Model file for the job. Use its own axes, mm. Coordinates: 2 decimals unless noted, no trailing zeros. Write each loop counter-clockwise with the first axis right and the second up, starting at its lowest first coordinate (ties: lowest second). Pieces come first, ordered by that corner, then holes. Notation, with made-up numbers: M 45,80 L 73,80 A23 ccw 73,91 Z; hole C 48.5,-38.5 d5. An arc over 180 degrees is marked long. Put each result on its own line as item: value. Start each with the question number.
Q1. Cut at A-A (y = 15). Write the cut outline in (x, z), then the cut area to 3 significant figures.
Q2. Cut at C-C (x = -7.75). Write the cut outline in (y, z), then the cut area to 3 significant figures.
Q3. Drill centre lines: line 1 along Z through (x, y) = (0.75, 28); line 2 along Z through (x, y) = (-5, 13.5); line 3 along X through (y, z) = (8.5, 35). Where is each one in solid material? Low to high.
Q4. Pull direction X, two halves, no side cores. Call faces 1 (the cylindrical face through (2.4, 15.2, 38.2)), 2 (the flat face through (0, 0, -1)), 3 (the flat face through (15, 15, 1)): pulls with the +X half, pulls with the -X half, needs draft (parallel to the pull), parting line crosses it, or undercut.
Q5. Cut at D-D (x = 2.5). Write the cut outline in (y, z), then the cut area to 3 significant figures.
Q6. Cut at B-B (z = -20). Write the cut outline in (x, y).
```python
from build123d import *

# Parameters (mm, degrees)
SKETCH1_W           = 30
SKETCH1_H           = 90
BOSS_EXTRUDE1_DEPTH = 30
SKETCH2_R           = 4
CUT_EXTRUDE1_DEPTH  = 62.846584384
SKETCH3_R           = 4
CUT_EXTRUDE2_DEPTH  = 57.124860802


with BuildPart() as part:
    # Sketch1 → Boss-Extrude1 (new body)
    with BuildSketch(Plane(origin=(0, 0, 0), x_dir=(1, 0, 0), z_dir=(0, 1, 0))):
        Rectangle(SKETCH1_W, SKETCH1_H)
    extrude(amount=BOSS_EXTRUDE1_DEPTH)

    # Sketch2 → Cut-Extrude1 (cut, through all)
    with BuildSketch(Plane.ZY.offset(15)):
        with Locations((-20, 15)):
            Circle(SKETCH2_R)
        with Locations((20, 15)):
            Circle(SKETCH2_R)
    extrude(amount=-CUT_EXTRUDE1_DEPTH, mode=Mode.SUBTRACT)

    # Sketch3 → Cut-Extrude2 (cut, through all)
    with BuildSketch(Plane(origin=(0, 30, 0), x_dir=(1, 0, 0), z_dir=(0, 1, 0))):
        with Locations(Location((0, 35, 0), (0, 0, 270))):
            Circle(SKETCH3_R)
        with Locations(Location((0, -35, 0), (0, 0, 90))):
            Circle(SKETCH3_R)
    extrude(amount=-CUT_EXTRUDE2_DEPTH, mode=Mode.SUBTRACT)


solid = part.part
```
Computed values:
1. outline: M -15,-45 L 15,-45 L 15,-24 L -15,-24 Z; M -15,-16 L 15,-16 L 15,16 L -15,16 Z; M -15,24 L 15,24 L 15,45 L -15,45 Z; hole C 0,-35 d8; hole C 0,35 d8
1. area: 2,120 mm2
2. outline: M 0,-45 L 30,-45 L 30,45 L 0,45 Z; hole C 15,-20 d8; hole C 15,20 d8
2. area: 2,600 mm2
3. line 1: -45 to -38.93, -31.07 to 31.07, 38.93 to 45
3. line 2: -45 to -23.71, -16.29 to 16.29, 23.71 to 45
3. line 3: -15 to -4, 4 to 15
4. face 1: undercut
4. face 2: needs draft
4. face 3: pulls with the +X half
5. outline: M 0,-45 L 30,-45 L 30,-38.12 L 0,-38.12 Z; M 0,-31.88 L 30,-31.88 L 30,31.88 L 0,31.88 Z; M 0,38.12 L 30,38.12 L 30,45 L 0,45 Z; hole C 15,-20 d8; hole C 15,20 d8
5. area: 2,220 mm2
6. outline: M -15,0 L 15,0 L 15,11 L -15,11 Z; M -15,19 L 15,19 L 15,30 L -15,30 Z
